Part print with two shaded views. Sizes in mm from the minimum x, y, z corner. A direction names the side the tool comes from. Round coordinates to 2 decimals unless told otherwise and drop trailing zeros. Loops run counter-clockwise (first coordinate to the right, second up) from the corner with the lowest first, then second, coordinate; pieces in that order, holes last. Notation, with made-up numbers: (-14.5, 56) -> (-3.5, 56) arc R24 ccw to (-3.5, 70) -> close; hole circle Ø6 at (74, 68). An arc over 180 degrees is marked (long way). Use a Markdown table: item, result. Add a question column.
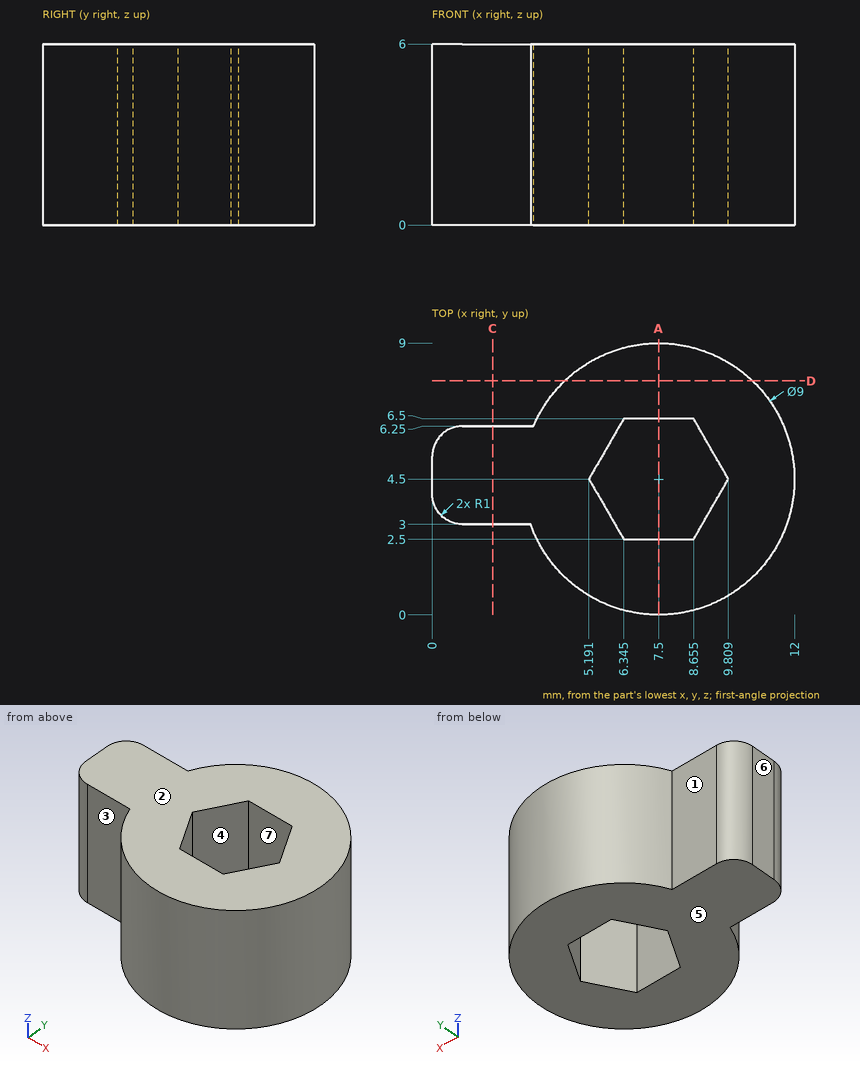
1) Cut at C-C on x = 2. Write the cut outline in (y, z).
2) Wall check: probe 1 along Y at (x, z) = (6, 4.4) (1 decimal); probe 2 along Y at (x, z) = (5.25, 4.1) (1 decimal); probe 3 along Y at (x, z) = (2.25, 3.2). Give the ranges that are in metal, low to high. Write a range as from..to.
3) Cut at A-A on x = 7.5. Write the cut outline in (y, z), and give its area (3 significant figures).
4) Tool access for the marked faces 1, 2, 3 and 4: list every direction of +Z, -Z, +X, -X, +Y, -Y with a clear straight run to the whole face (end or side of a thin tool).
5) Cut at D-D on y = 7.75. Write the cut outline in (x, z).
6) Pin check, flat tips, straight feed: pin 1 Ø3 at (y, z) = (1, 5) entering from +X; pin 2 Ø1.8 at (x, z) = (1.5, 4.5) entering from -Y; pin 3 Ø0.7 at (x, z) = (1.5, 2) entering from +Y. Stop position of each tip, or through.
7) Pull direction X, two halves, no side cores. Call the marked faces 5, 6 and 7: +X half, -X half, draft (parallel to the pull), parting line (faces both ways), or undercut.
Established:
| question | item | result |
|---|---|---|
| 1 | outline | (3, 0) -> (6.25, 0) -> (6.25, 6) -> (3, 6) -> close |
| 2 | probe 1 | y = 0.3..3.1, 5.9..8.7 |
| 2 | probe 2 | y = 0.6..4.4, 4.6..8.4 |
| 2 | probe 3 | y = 3..6.25 |
| 3 | outline | (0, 0) -> (2.5, 0) -> (2.5, 6) -> (0, 6) -> close; (6.5, 0) -> (9, 0) -> (9, 6) -> (6.5, 6) -> close |
| 3 | area | 30.0 mm^2 |
| 4 | face 1 | +Z, -Z, -X, +Y |
| 4 | face 2 | +Z, +X, -X, +Y, -Y |
| 4 | face 3 | +Z, -Z, -X, -Y |
| 4 | face 4 | +Z, -Z |
| 5 | outline | (4.39, 0) -> (10.61, 0) -> (10.61, 6) -> (4.39, 6) -> close |
| 6 | pin 1 | stops at x = 11.53 |
| 6 | pin 2 | stops at y = 3 |
| 6 | pin 3 | stops at y = 6.25 |
| 7 | face 5 | draft |
| 7 | face 6 | -X half |
| 7 | face 7 | undercut |
